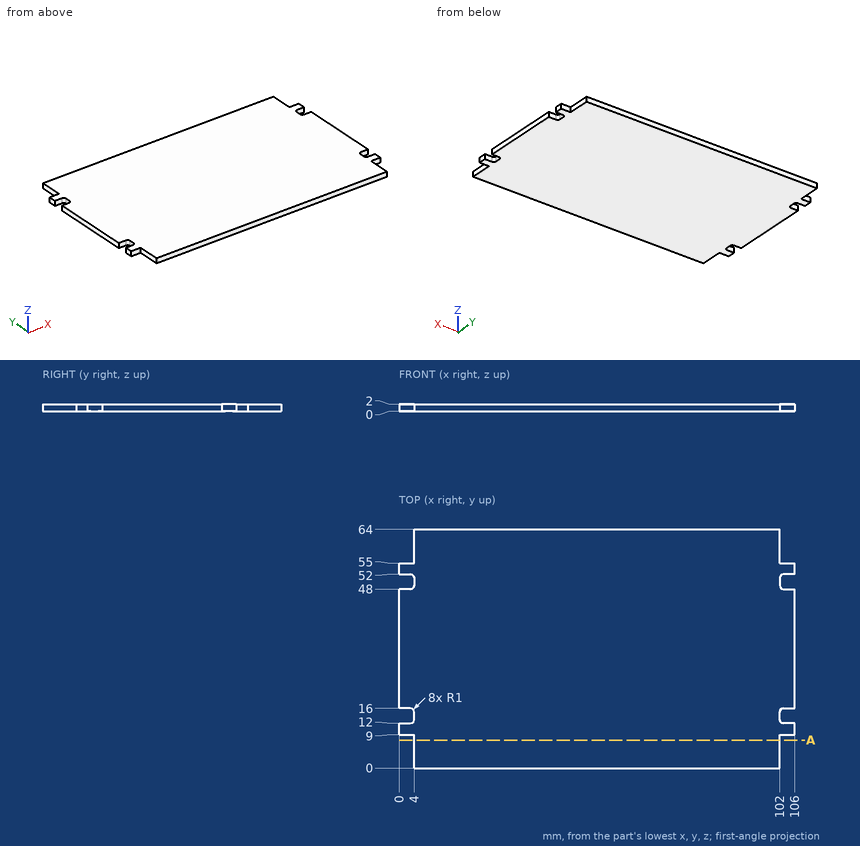
Check sheet for the drawn part. Datum: minimum x, y, z corner. Units: mm. Coordinates: 2 decimals unless noted, no trailing zeros. Write each loop counter-clockwise with the first axis right and the second up, starting at its lowest first coordinate (ties: lowest second). Pieces come first, ordered by that corner, then holes. Notation, with made-up numbers: (-20, 7.25) - (11, 7.25) arc R15 ccw to (11, 17.25) - close; hole circle Ø11 at (8.25, -24.75). An arc over 180 degrees is marked (long way). Answer as a JSON object with one key per item and string values.
(1) Thickness scan on line 1 along X through (y, z) = (13.5, 0.95); line 2 along X through (y, z) = (48.5, 0.1). Record the ranges inside material, lowest first.
Report:
{"line 1": "4 to 102", "line 2": "3.87 to 102.13"}
(2) Gauge pin test, flat ends, axial feed: pin 1 Ø0.6 at (x, z) = (2.5, 1.5) entering from +Y; pin 2 Ø0.6 at (y, z) = (50.5, 1) entering from -X; pin 3 Ø1 at (x, z) = (1, 1) entering from -Y; pin 4 Ø3 at (x, y) = (35, 17.5) entering from -Z. Record the tip position at first contact, or that the pin passes through.
Report:
{"pin 1": "y = 55", "pin 2": "x = 4", "pin 3": "y = 9", "pin 4": "z = 0"}
(3) Cross-section at A-A on y = 7.5. Record the cut outline in (x, z).
Report:
{"outline": "(4, 0) - (102, 0) - (102, 2) - (4, 2) - close"}
